The listing builds one solid part. Answer for the finished solid, in the listing's coordinates (mm). Give positions to 0.01 mm unless a question says otherwise; leave off trailing zeros. Order: outer loops, then holes, each group sorted by start corner. A loop starts at its lowest first (then second) coordinate and runs counter-clockwise, first axis right, second up. Notation, with made-up numbers: (19, 66) - (75, 66) arc R22 ccw to (75, 74) - close; hole circle Ø6 at (-33.5, 45.25). An arc over 180 degrees is marked (long way). Use a Markdown table: item, result. Add a question column.
1) Find section B-B, the plane z = -32. Determine the outline of the cut face in (x, y).
2) Straight lines are drawn through the part: line 1 (X direction, y = 0.65, z = -32); line 2 (X direction, y = 0.5, z = 16.5). For each, find the intervals that lie inside material, in ascending order.
3) Find section A-A, the plane x = 13. Determine the outline of the cut face in (y, z).
4) Find section D-D, the plane z = 13. Determine the outline of the cut face in (x, y), plus the area to 3 significant figures.
5) Find section C-C, the plane y = 0.25. Determine the outline of the cut face in (x, z).
from build123d import *

# Parameters (mm, degrees)
SKETCH_1_W      = 64
SKETCH_1_H      = 74
SKETCH_1_R      = 1.5
SKETCH_1_R_2    = 11
EXTRUDE_1_DEPTH = 1.6
FILLET_1_R      = 2


with BuildPart() as part:
    # 草图1 → 凸台-拉伸1 (new body)
    with BuildSketch(Plane(origin=(0, 0, 0), x_dir=(1, 0, 0), z_dir=(0, 1, 0))):
        Rectangle(SKETCH_1_W, SKETCH_1_H)
        with Locations(Location((26, 32, 0), (0, 0, 270))):
            Circle(SKETCH_1_R, mode=Mode.SUBTRACT)
        with Locations(Location((-26, 32, 0), (0, 0, 90))):
            Circle(SKETCH_1_R, mode=Mode.SUBTRACT)
        with Locations(Location((13, -13, 0), (0, 0, 270))):
            Circle(SKETCH_1_R_2, mode=Mode.SUBTRACT)
        with Locations(Location((26, -32, 0), (0, 0, 90))):
            Circle(SKETCH_1_R, mode=Mode.SUBTRACT)
        with Locations(Location((-26, -32, 0), (0, 0, 270))):
            Circle(SKETCH_1_R, mode=Mode.SUBTRACT)
    extrude(amount=EXTRUDE_1_DEPTH)

    # 圆角1
    fillet_1_edges = [part.edges().sort_by_distance(p)[0] for p in [
        (32, 0.8, 37),
        (-32, 0.8, 37),
        (-32, 0.8, -37),
        (32, 0.8, -37),
    ]]
    fillet(fillet_1_edges, radius=FILLET_1_R)


solid = part.part
The answers:
| question | item | result |
|---|---|---|
| 1 | outline | (-32, 0) - (-27.5, 0) - (-27.5, 1.6) - (-32, 1.6) - close; (-24.5, 0) - (24.5, 0) - (24.5, 1.6) - (-24.5, 1.6) - close; (27.5, 0) - (32, 0) - (32, 1.6) - (27.5, 1.6) - close |
| 2 | line 1 | -32 to -27.5, -24.5 to 24.5, 27.5 to 32 |
| 2 | line 2 | -32 to 2.57, 23.43 to 32 |
| 3 | outline | (0, -37) - (1.6, -37) - (1.6, 2) - (0, 2) - close; (0, 24) - (1.6, 24) - (1.6, 37) - (0, 37) - close |
| 4 | outline | (-32, 0) - (2, 0) - (2, 1.6) - (-32, 1.6) - close; (24, 0) - (32, 0) - (32, 1.6) - (24, 1.6) - close |
| 4 | area | 67.2 mm2 |
| 5 | outline | (-32, -35) arc R2 ccw to (-30, -37) - (30, -37) arc R2 ccw to (32, -35) - (32, 35) arc R2 ccw to (30, 37) - (-30, 37) arc R2 ccw to (-32, 35) - close; hole circle Ø3 at (-26, -32); hole circle Ø3 at (-26, 32); hole circle Ø22 at (13, 13); hole circle Ø3 at (26, -32); hole circle Ø3 at (26, 32) |
